from build123d import *

# Parameters (mm, degrees)
F0_R           = 2.54
F0_W           = 43.18
F0_H           = 43.18
F0_W_2         = 8.89
F0_W_3         = 11.43
F0_H_2         = 11.43
F1_DEPTH       = 2.54
F2_DEPTH       = 6.35
F3_D           = 3.302
F5_D           = 3.175
F5_CSINK_D     = 6.858
F5_CSINK_ANGLE = 90


with BuildPart() as f1:
    # F0 (on Top) → F1 (new body)
    with BuildSketch(Plane.XY):
        Polygon((30.48, 21.59), (30.48, 30.48), (5.715, 30.48), (-5.715, 30.48), (-30.48, 30.48), (-30.48, 21.59), (-30.48, -21.59), (-30.48, -30.48), (-5.715, -30.48), (5.715, -30.48), (30.48, -30.48), (30.48, -21.59), align=None)
        with Locations((-25.4, -25.4)):
            Circle(F0_R, mode=Mode.SUBTRACT)
        with Locations((25.4, -25.4)):
            Circle(F0_R, mode=Mode.SUBTRACT)
        with Locations((-25.4, 25.4)):
            Circle(F0_R, mode=Mode.SUBTRACT)
        Rectangle(F0_W, F0_H, mode=Mode.SUBTRACT)
        with Locations((25.4, 25.4)):
            Circle(F0_R, mode=Mode.SUBTRACT)
        Polygon((-30.48, 21.59), (-30.48, 30.48), (-80.01, 30.48), (-91.44, 30.48), (-91.44, 21.59), (-82.55, 21.59), align=None)
        with Locations((-86.36, 25.4)):
            Circle(F0_R, mode=Mode.SUBTRACT)
        with Locations((-35.56, 25.4)):
            Circle(F0_R, mode=Mode.SUBTRACT)
        with Locations((-86.995, 0)):
            Rectangle(F0_W_2, F0_H)
        Polygon((-30.48, -30.48), (-30.48, -21.59), (-82.55, -21.59), (-91.44, -21.59), (-91.44, -30.48), (-80.01, -30.48), align=None)
        with Locations((-86.36, -25.4)):
            Circle(F0_R, mode=Mode.SUBTRACT)
        with Locations((-35.56, -25.4)):
            Circle(F0_R, mode=Mode.SUBTRACT)
        Polygon((80.01, 30.48), (30.48, 30.48), (30.48, 21.59), (82.55, 21.59), (91.44, 21.59), (91.44, 30.48), align=None)
        with Locations((35.56, 25.4)):
            Circle(F0_R, mode=Mode.SUBTRACT)
        with Locations((86.36, 25.4)):
            Circle(F0_R, mode=Mode.SUBTRACT)
        Polygon((82.55, -21.59), (30.48, -21.59), (30.48, -30.48), (80.01, -30.48), (91.44, -30.48), (91.44, -21.59), align=None)
        with Locations((35.56, -25.4)):
            Circle(F0_R, mode=Mode.SUBTRACT)
        with Locations((86.36, -25.4)):
            Circle(F0_R, mode=Mode.SUBTRACT)
        with Locations((86.995, 0)):
            Rectangle(F0_W_2, F0_H)
        with Locations((-85.725, 36.195)):
            Rectangle(F0_W_3, F0_H_2)
        with Locations((85.725, 36.195)):
            Rectangle(F0_W_3, F0_H_2)
        with Locations((85.725, -36.195)):
            Rectangle(F0_W_3, F0_H_2)
        with Locations((-85.725, -36.195)):
            Rectangle(F0_W_3, F0_H_2)
        with Locations((0, 36.195)):
            Rectangle(F0_W_3, F0_H_2)
        with Locations((0, -36.195)):
            Rectangle(F0_W_3, F0_H_2)
    extrude(amount=F1_DEPTH)

    # F0 (on Top) → F2 (join)
    with BuildSketch(Plane.XY):
        with Locations((-25.4, 25.4)):
            Circle(F0_R)
        with Locations((25.4, 25.4)):
            Circle(F0_R)
        with Locations((25.4, -25.4)):
            Circle(F0_R)
        with Locations((-25.4, -25.4)):
            Circle(F0_R)
        with Locations((-86.36, 25.4)):
            Circle(F0_R)
        with Locations((-86.36, -25.4)):
            Circle(F0_R)
        with Locations((-35.56, 25.4)):
            Circle(F0_R)
        with Locations((-35.56, -25.4)):
            Circle(F0_R)
        with Locations((35.56, -25.4)):
            Circle(F0_R)
        with Locations((86.36, -25.4)):
            Circle(F0_R)
        with Locations((86.36, 25.4)):
            Circle(F0_R)
        with Locations((35.56, 25.4)):
            Circle(F0_R)
    extrude(amount=F2_DEPTH)

    # F3 (through all)
    with Locations(Plane(origin=(0, 0, 0), x_dir=(1, 0, 0), z_dir=(0, 0, -1))):
        with Locations((-25.4, 25.4), (25.4, 25.4), (25.4, -25.4), (-25.4, -25.4), (-86.36, 25.4), (-35.56, 25.4), (-86.36, -25.4), (-35.56, -25.4), (35.56, 25.4), (86.36, 25.4), (35.56, -25.4), (86.36, -25.4)):
            Hole(F3_D / 2)

    # F5 (through all)
    with Locations(Plane.XY.offset(2.54)):
        with Locations((-85.725, 36.195), (-85.725, -36.195), (85.725, -36.195), (85.725, 36.195), (0, 36.195), (0, -36.195)):
            CounterSinkHole(F5_D / 2, F5_CSINK_D / 2, counter_sink_angle=F5_CSINK_ANGLE)


solid = f1.part
Build history of the part. All positions in model axes, mm. A direction names the side the tool comes from. Round coordinates to 2 decimals unless told otherwise and drop trailing zeros. Write each loop counter-clockwise with the first axis right and the second up, starting at its lowest first coordinate (ties: lowest second). Pieces come first, ordered by that corner, then holes. Notation, with made-up numbers: M -27,-5.5 L 19,-5.5 A29 ccw 19,16.5 Z; hole C 66.5,79 d7. An arc over 180 degrees is marked long. Answer as a JSON object with one key per item and string values. Group by question number.
(1) Cut at A-A (x = -25.4). Give the cut face in (y, z), and give its area (3 significant figures).
(2) Drill centre lines: L1, parallel to X at y = 4, z = 2; L2, parallel to Y at x = 35.56, z = 3.5. Where is each one in solid material? Low to high.
(3) Cut at D-D (y = -25.4). Give the number of separate pieces and of enclosed holes in the cut face, and give its area (3 significant figures).
(4) Mould opens along Y. For faces 1 (the flat face through (-36.2, -27.1, 6.35)), 2 (the cylindrical face through (34.67, -26.79, 3.22)) say: pulls with the +Y half, pulls with the -Y half, needs draft (parallel to the pull), parting line crosses it, or undercut.
(5) Cut at B-B (y = -16). Give the cut face in (x, z).
(6) Which spindle directions (+Z, -Z, +X, -X, +Y, -Y) get a long thin tool onto all of the face, cutting with end or side? Do faces 3 (the cylindrical face through (-83.937, 26.163, 4.418)), 4 (the flat face through (24.8, -27.1, 6.35)). Say none if no direction does.
(7) Flat gauge pins, fed straight in: pin 1 (3 mm diameter, centred on x = 50.5, z = 1.5, fed in from -Y); pin 2 (3.5 mm diameter, centred on x = -85.725, y = 36.195, fed in from +Z). Where does each tip first touch, or does it go through?
(8) Cut at C-C (x = -68.5). Give the cut face in (y, z), and give its area (3 significant figures).
Responses:
{
 "1": {"outline": "M -30.48,0 L -27.05,0 L -27.05,6.35 L -27.94,6.35 L -27.94,2.54 L -30.48,2.54 Z; M -23.75,0 L 23.75,0 L 23.75,6.35 L 22.86,6.35 L 22.86,2.54 L -22.86,2.54 L -22.86,6.35 L -23.75,6.35 Z; M 27.05,0 L 30.48,0 L 30.48,2.54 L 27.94,2.54 L 27.94,6.35 L 27.05,6.35 Z", "area": "152 mm2"},
 "2": {"L1": "x = -91.44 to -82.55, -30.48 to -21.59, 21.59 to 30.48, 82.55 to 91.44", "L2": "y = -27.94 to -27.05, -23.75 to -22.86, 22.86 to 23.75, 27.05 to 27.94"},
 "3": {"separate pieces": "7", "enclosed holes": "0", "area": "455 mm2"},
 "4": {"face 1": "needs draft", "face 2": "undercut"},
 "5": {"outline": "M -91.44,0 L -82.55,0 L -82.55,2.54 L -91.44,2.54 Z; M -30.48,0 L -21.59,0 L -21.59,2.54 L -30.48,2.54 Z; M 21.59,0 L 30.48,0 L 30.48,2.54 L 21.59,2.54 Z; M 82.55,0 L 91.44,0 L 91.44,2.54 L 82.55,2.54 Z"},
 "6": {"face 3": "+Z", "face 4": "+Z, +X, -X, +Y, -Y"},
 "7": {"pin 1": "stops at y = -30.48", "pin 2": "stops at z = 0.86"},
 "8": {"outline": "M -30.48,0 L -21.59,0 L -21.59,2.54 L -30.48,2.54 Z; M 21.59,0 L 30.48,0 L 30.48,2.54 L 21.59,2.54 Z", "area": "45.2 mm2"}
}
